from build123d import *

# Parameters (mm, degrees)
F1_DEPTH = 26
F3_DEPTH = 10.001
F4_R     = 12.99999
F5_R     = 7
F6_DEPTH = 4.4
F7_R     = 3.3
F8_DEPTH = 53.801


# Not quite as in the source:
# - a fillet or chamfer is up to 0.001 mm smaller than in the source, because OpenCascade refuses the exact size


with BuildPart() as f1:
    # F0 (on Front) → F1 (new body)
    with BuildSketch(Plane.XZ):
        with BuildLine():
            Line((-38.8, 0), (0, 0))
            Line((0, 0), (11.9, 20.6114046101))
            Line((11.9, 20.6114046101), (14.1603821252, 25.0713006457))
            Line((14.1603821252, 25.0713006457), (18.7301270189, 22.441531629))
            Line((18.7301270189, 22.441531629), (31.7205080757, 14.941531629))
            Line((31.7205080757, 14.941531629), (36.7205080757, 23.6017856668))
            Line((36.7205080757, 23.6017856668), (19.4, 33.6017856668))
            Line((19.4, 33.6017856668), (10.7397459622, 38.6017856668))
            Line((10.7397459622, 38.6017856668), (-4.3301270189, 12.5))
            ThreePointArc((-4.3301270189, 12.5), (-6.1602540378, 10.6698729811), (-8.6602540378, 10))
            Line((-8.6602540378, 10), (-33.8, 10))
            ThreePointArc((-33.8, 10), (-37.3355339059, 8.5355339059), (-38.8, 5))
            Line((-38.8, 5), (-38.8, 0))
        make_face()
    extrude(amount=F1_DEPTH)

    # F2 (on face) → F3 (cut, through all)
    with BuildSketch(Plane.XY.offset(10)):
        with BuildLine():
            ThreePointArc((-28.7603622502, -15.99973813), (-26.6647115828, -15.1072596839), (-25.8, -13))
            ThreePointArc((-25.8, -13), (-26.6495430639, -10.9082220563), (-28.7170233106, -10.0011477414))
            ThreePointArc((-28.7170233106, -10.0011477414), (-31.7993750812, -12.9387699222), (-28.839480247, -15.9997402071))
            Line((-28.839480247, -15.9997402071), (-28.7603622502, -15.99973813))
        make_face()
        with BuildLine():
            ThreePointArc((-28.7170233106, -10.0011477414), (-26.6495430639, -10.9082220563), (-25.8, -13))
            ThreePointArc((-25.8, -13), (-26.6647115828, -15.1072596839), (-28.7603622502, -15.99973813))
            Line((-28.7603622502, -15.99973813), (-16.7999212569, -15.9994241356))
            ThreePointArc((-16.7999212569, -15.9994241356), (-19.7994241345, -13.0001113407), (-16.8001439382, -10.0005758668))
            Line((-16.8001439382, -10.0005758668), (-28.7170233106, -10.0011477414))
        make_face()
        with BuildLine():
            ThreePointArc((-28.839480247, -15.9997402071), (-28.7999212418, -15.999999999), (-28.7603622502, -15.99973813))
            Line((-28.7603622502, -15.99973813), (-28.839480247, -15.9997402071))
        make_face()
        with BuildLine():
            ThreePointArc((-13.8005758634, -13), (-14.6791377438, -10.8790359641), (-16.8001439382, -10.0005758668))
            ThreePointArc((-16.8001439382, -10.0005758668), (-19.7994241345, -13.0001113407), (-16.7999212569, -15.9994241356))
            ThreePointArc((-16.7999212569, -15.9994241356), (-14.6790590136, -15.1208853066), (-13.8005758634, -13))
        make_face()
    extrude(amount=-F3_DEPTH, mode=Mode.SUBTRACT)

    # F4 (radius 13 in the source; OpenCascade refuses exactly that, so slightly less here)
    f4_edges = [f1.edges().sort_by_distance(p)[0] for p in [
        (34.220508, -26, 19.271659),
        (34.220508, 0, 19.271659),
    ]]
    fillet(f4_edges, radius=F4_R)

    # F5 (on face) → F6 (cut)
    with BuildSketch(Plane(origin=(19.4, 0, 33.6017856668), x_dir=(0.8660254038, 0, -0.5), z_dir=(0.5, 0, 0.8660254038))):
        with Locations((7, -13)):
            Circle(F5_R)
    extrude(amount=-F6_DEPTH, mode=Mode.SUBTRACT)

    # F7 (on face) → F8 (cut, through all)
    with BuildSketch(Plane(origin=(17.2, 0, 29.7912738902), x_dir=(0.8660254038, 0, -0.5), z_dir=(0.5, 0, 0.8660254038))):
        with Locations((7, -13)):
            Circle(F7_R)
    extrude(amount=-F8_DEPTH, mode=Mode.SUBTRACT)


solid = f1.part
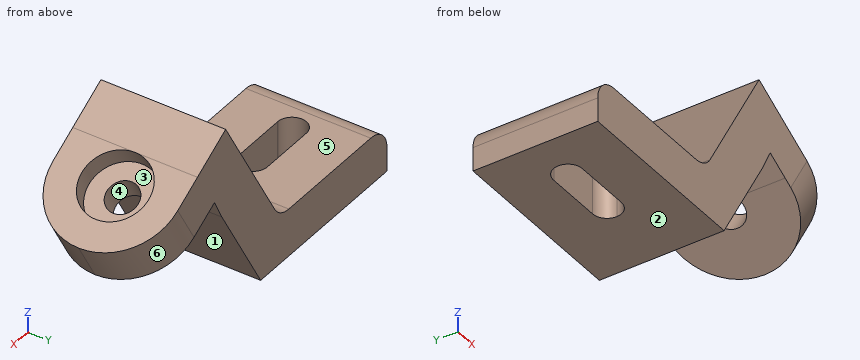
For this review, take the finished solid that the model builds, in its own axes (mm). Face numbers are marked on the shaded views. A direction names the side the tool comes from. Coordinates: 2 decimals unless noted, no trailing zeros. Loops run counter-clockwise (first coordinate to the right, second up) from the corner with the lowest first, then second, coordinate; pieces in that order, holes last. Notation, with made-up numbers: (-33.5, 65.25) -> (-21.5, 65.25) arc R18 ccw to (-21.5, 82.25) -> close; hole circle Ø1 at (35.25, 74.5). An arc over 180 degrees is marked (long way). Write each question's results on one line, items separated by ' | '.
Q1. To check wall thickness, follow line 1 along Y through (x, z) = (-23.5, 3); line 2 along Z through (x, y) = (-9, -11.25); line 3 along Z through (x, y) = (0, -2). State the ranges of each line that lie inside material, in increasing order. Write a range as [from, to].
Taken from the geometry:
line 1: [-26, -16], [-10, 0] | line 2: [0, 10] | line 3: [0, 20]
Q2. Add section B-B, the plane z = 6. State the section outline as (x, y) points.
Taken from the geometry:
outline: (-38.7, -26) -> (3.46, -26) -> (3.46, 0) -> (-38.7, 0) -> close; hole (-28.76, -16) -> (-16.8, -16) arc R3 ccw to (-16.8, -10) -> (-28.72, -10) arc R3 ccw (long way) to start
Q3. Mouldability with a two-part tool opening along Y and no side actions: class the marked faces 4, 5 and 6 as +Y half, -Y half, draft (parallel to the pull), parting line (faces both ways), or undercut.
Taken from the geometry:
face 4: undercut | face 5: draft | face 6: +Y half
Q4. Add section C-C, the plane y = -22.5. State the section outline as (x, z) points.
Taken from the geometry:
outline: (-38.8, 0) -> (0, 0) -> (11.9, 20.61) -> (14.16, 25.07) -> (18.73, 22.44) -> (28.15, 17) -> (33.15, 25.66) -> (10.74, 38.6) -> (-4.33, 12.5) arc R5 cw to (-8.66, 10) -> (-33.8, 10) arc R5 ccw to (-38.8, 5) -> close
Q5. Add section A-A, the plane y = -14. State the section outline as (x, z) points, then the cut area to 3 significant figures.
Taken from the geometry:
outline: (-38.8, 0) -> (-31.63, 0) -> (-31.63, 10) -> (-33.8, 10) arc R5 ccw to (-38.8, 5) -> close; (-13.97, 0) -> (0, 0) -> (11.9, 20.61) -> (14.16, 25.07) -> (17.74, 23.01) -> (20.54, 27.86) -> (17.26, 29.76) -> (19.46, 33.57) -> (10.74, 38.6) -> (-4.33, 12.5) arc R5 cw to (-8.66, 10) -> (-13.97, 10) -> close; (23.19, 19.87) -> (31.69, 14.96) -> (36.69, 23.62) -> (31.46, 26.64) -> (29.26, 22.83) -> (25.99, 24.72) -> close | area: 640 mm²
Q6. Machinability: for the marked faces 1, 2 and 3, which of the approach directions +Z, -Z, +X, -X, +Y, -Y give a long, thin tool a straight path to every point of the face, cutting with its end or side? Answer none if there is none.
Taken from the geometry:
face 1: -Z, +Y, -Y | face 2: -Z, +X, -X, +Y, -Y | face 3: none
Q7. For pin 1 Ø3 at (y, z) = (-4.5, 9.5) entering from +X; pin 2 Ø10 at (y, z) = (-17, 13) entering from -X; pin 3 Ø4 at (x, y) = (0, -20.5) entering from +Z; pin 4 Ø6 at (x, z) = (2, 30.5) entering from +Y (3 decimals), all flat-tipped, find the tip position at first contact; note any pin that passes through.
Taken from the geometry:
pin 1: x = 6.35 | pin 2: x = -37.8 | pin 3: z = 23.46 | pin 4: through
Q8. Add section D-D, the plane x = 4.5. State the section outline as (y, z) points, then the cut area to 3 significant figures.
Taken from the geometry:
outline: (-26, 7.79) -> (0, 7.79) -> (0, 27.79) -> (-26, 27.79) -> close | area: 520 mm²
